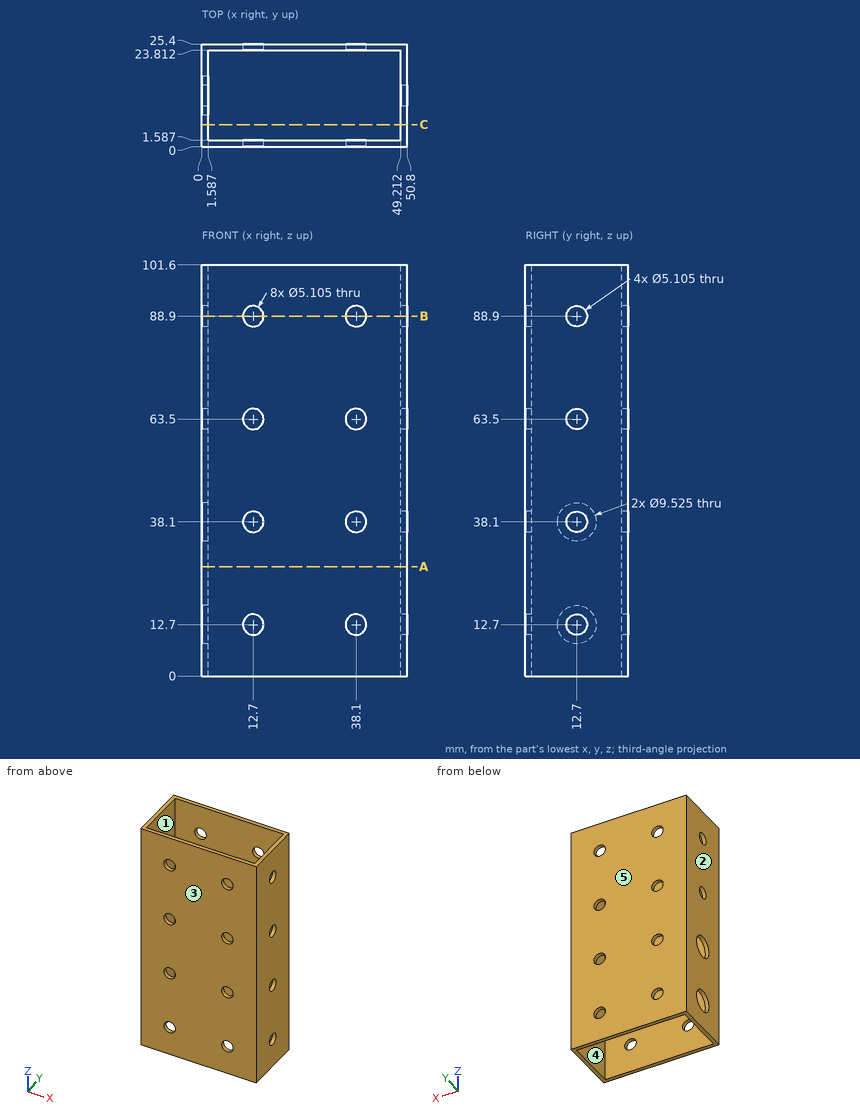
Here's the drawing with two shaded views (mm, measured from the low corner). I have some questions. A direction names the side the tool comes from. Coordinates: 2 decimals unless noted, no trailing zeros. Loops run counter-clockwise (first coordinate to the right, second up) from the corner with the lowest first, then second, coordinate; pieces in that order, holes last. Notation, with made-up numbers: (9, 18.25) -> (43, 18.25) arc R13 ccw to (43, 35.25) -> close; hole circle Ø9 at (-29.75, 60). An arc over 180 degrees is marked (long way). Answer in a Markdown table with one row per item.
(1) Imagine slicing it at C-C (y = 5.5). List the corners of the cut face in (x, z) for me.
Results found:
| item | result |
|---|---|
| outline | (0, 0) -> (1.59, 0) -> (1.59, 101.6) -> (0, 101.6) -> close; (49.21, 0) -> (50.8, 0) -> (50.8, 101.6) -> (49.21, 101.6) -> close |
(2) For the marked faces 4 and 5, which set-ups out of +Z, -Z, +X, -X, +Y, -Y let a thin tool reach every point of the face, with its end or its side?
Results found:
| item | result |
|---|---|
| face 4 | +Z, -Z |
| face 5 | +Z, -Z, +X, -X, +Y |
(3) Will these pins go through, and if not, where does the flat tip stop? pin 1 Ø3 at (y, z) = (12.7, 12.7) entering from -X; pin 2 Ø8.5 at (y, z) = (12.7, 38.1) entering from -X.
Results found:
| item | result |
|---|---|
| pin 1 | passes through |
| pin 2 | stops at x = 49.21 |
(4) Thinking about a two-plate mould opening in X: for the marked faces 1, 2 and 3, which applies, released by +X, released by -X, zero draft, split by the parting line, or undercut?
Results found:
| item | result |
|---|---|
| face 1 | undercut |
| face 2 | released by -X |
| face 3 | zero draft |
(5) Imagine slicing it at A-A (z = 27). List the corners of the cut face in (x, y) for me, plus the area to 3 significant figures.
Results found:
| item | result |
|---|---|
| outline | (0, 0) -> (50.8, 0) -> (50.8, 25.4) -> (0, 25.4) -> close; hole (1.59, 1.59) -> (49.21, 1.59) -> (49.21, 23.81) -> (1.59, 23.81) -> close |
| area | 232 mm^2 |
(6) If I drill on probe 1 along Z at (x, y) = (12.7, 24.35); probe 2 along Z at (x, y) = (0.5, 12.7); probe 3 along X at (y, z) = (21.5, 83.5), over which ranges is the centre line in solid material (lowest first)?
Results found:
| item | result |
|---|---|
| probe 1 | z = 0 to 10.15, 15.25 to 35.55, 40.65 to 60.95, 66.05 to 86.35, 91.45 to 101.6 |
| probe 2 | z = 0 to 7.94, 17.46 to 33.34, 42.86 to 60.95, 66.05 to 86.35, 91.45 to 101.6 |
| probe 3 | x = 0 to 1.59, 49.21 to 50.8 |
(7) Imagine slicing it at B-B (z = 88.9). Give the number of separate pieces and of enclosed holes in the cut face, plus the area to 3 significant figures.
Results found:
| item | result |
|---|---|
| separate pieces | 6 |
| enclosed holes | 0 |
| area | 183 mm^2 |
